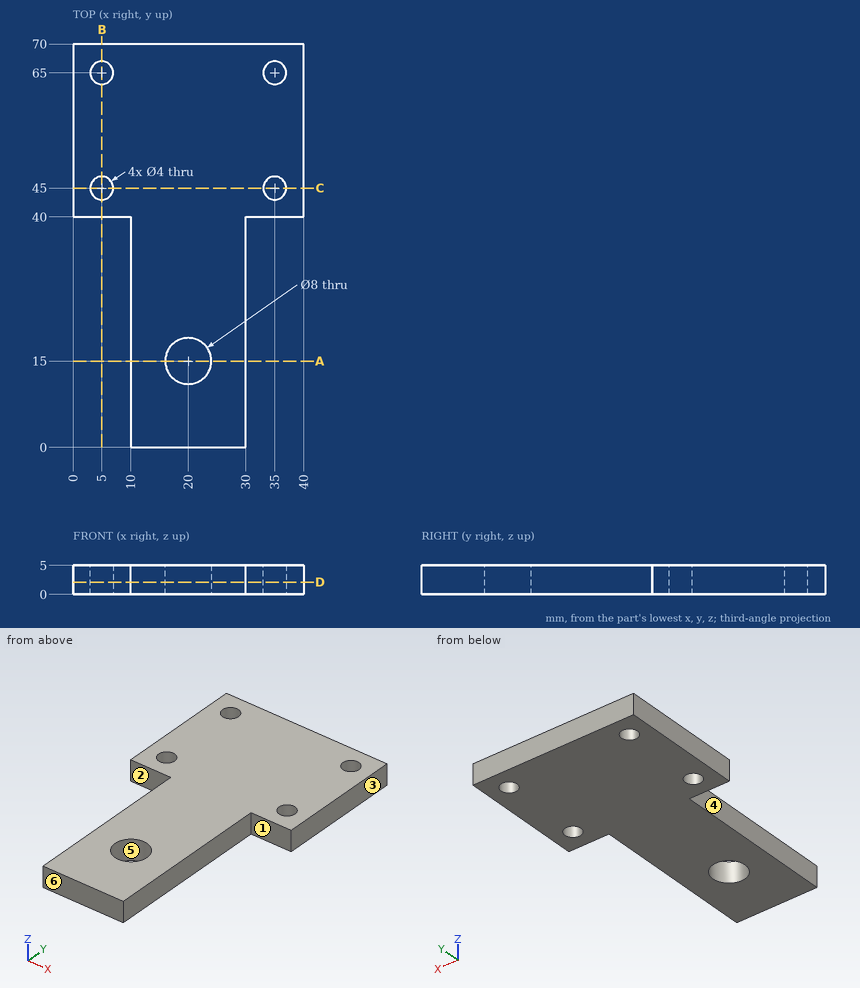
Verification items for this drawing (mm, ordinates from the low corner). A direction names the side the tool comes from. Coordinates: 2 decimals unless noted, no trailing zeros. Order: outer loops, then holes, each group sorted by start corner. A loop starts at its lowest first (then second) coordinate and runs counter-clockwise, first axis right, second up.
Q1. Sectioned sample at D-D on z = 2.1. Record the cut outline in (x, y).
Reply:
outline: (0, 40) - (10, 40) - (10, 0) - (30, 0) - (30, 40) - (40, 40) - (40, 70) - (0, 70) - close; hole circle Ø4 at (5, 45); hole circle Ø4 at (5, 65); hole circle Ø8 at (20, 15); hole circle Ø4 at (35, 45); hole circle Ø4 at (35, 65)
Q2. Thickness scan on probe 1 along Y at (x, z) = (35, 3.1); probe 2 along X at (y, z) = (65, 2.55); probe 3 along Y at (x, z) = (20, 1.15). Record the ranges inside material, lowest first.
Reply:
probe 1: y = 40 to 43, 47 to 63, 67 to 70
probe 2: x = 0 to 3, 7 to 33, 37 to 40
probe 3: y = 0 to 11, 19 to 70
Q3. Sectioned sample at A-A on y = 15. Record the cut outline in (x, z).
Reply:
outline: (10, 0) - (16, 0) - (16, 5) - (10, 5) - close; (24, 0) - (30, 0) - (30, 5) - (24, 5) - close
Q4. Depth check by flat-ended pin: pin 1 Ø7 at (x, y) = (20, 15) entering from +Z; pin 2 Ø1 at (y, z) = (13, 0.5) entering from +X. Enter the tip coordinate at first touch or a pass-through.
Reply:
pin 1: passes through
pin 2: stops at x = 30
Q5. Tool access check on the marked faces 1, 2 and 3. Record the directions out of +Z, -Z, +X, -X, +Y, -Y that give a thin tool (end or side, any length) a straight path to the whole face; none if there is none.
Reply:
face 1: +Z, -Z, +X, -Y
face 2: +Z, -Z, -X, -Y
face 3: +Z, -Z, +X, +Y, -Y
Q6. Sectioned sample at C-C on y = 45. Record the cut outline in (x, z), and give its area (3 significant figures).
Reply:
outline: (0, 0) - (3, 0) - (3, 5) - (0, 5) - close; (7, 0) - (33, 0) - (33, 5) - (7, 5) - close; (37, 0) - (40, 0) - (40, 5) - (37, 5) - close
area: 160 mm2
Q7. Sectioned sample at B-B on x = 5. Record the cut outline in (y, z).
Reply:
outline: (40, 0) - (43, 0) - (43, 5) - (40, 5) - close; (47, 0) - (63, 0) - (63, 5) - (47, 5) - close; (67, 0) - (70, 0) - (70, 5) - (67, 5) - close
Q8. Draft check along Y on the marked faces 4, 5 and 6. Enter one of: released by +Y, released by -Y, zero draft, split by the parting line, or undercut.
Reply:
face 4: zero draft
face 5: undercut
face 6: released by -Y
